Geometry: final body of the model. Coordinates: model frame, mm. Face numbers are marked on the shaded views. A direction names the side the tool comes from. Round coordinates to 2 decimals unless told otherwise and drop trailing zeros. Write each loop counter-clockwise with the first axis right and the second up, starting at its lowest first coordinate (ties: lowest second). Pieces come first, ordered by that corner, then holes. Notation, with made-up numbers: M 48.5,48 L 53.5,48 A19 cw 53.5,70 Z; hole C 67.5,5 d5. An arc over 180 degrees is marked long. Put each result on its own line as item: value. Start each with the question number.
Autodesk Inventor part; units mm, degrees
ref_plane "YZ Plane" through (0, 0, 0) normal (1, 0, 0) x (0, 1, 0)
ref_plane "XZ Plane" through (0, 0, 0) normal (0, 1, 0) x (-1, 0, 0)
ref_plane "XY Plane" through (0, 0, 0) normal (0, 0, 1) x (1, 0, 0)
sketch "Sketch1" plane through (0, 0, 0) normal (0, 0, 1) x (1, 0, 0)
  circle A0 centre (0, 0) radius 14.2875
  circle A1 centre (0, 0) radius 6.35
  dimension "d0" = 28.575
  dimension "d1" = 12.7
extrude "Extrusion1" add sketch "Sketch1" along normal blind 7.7724
sketch "Sketch2" plane through (0, 0, 0) normal (0, 0, -1) x (-1, 0, 0)
  circle A0 centre (0, 0) radius 15.5575
  circle A1 centre (0, 0) radius 14.2875
  circle A2 centre (0, 0) radius 6.35
  dimension "d4" = 31.115
  dimension "d5" = 12.7
extrude "Extrusion2" add sketch "Sketch2" along normal blind 1.524 contours A0 | A1
properties part number "bearing"
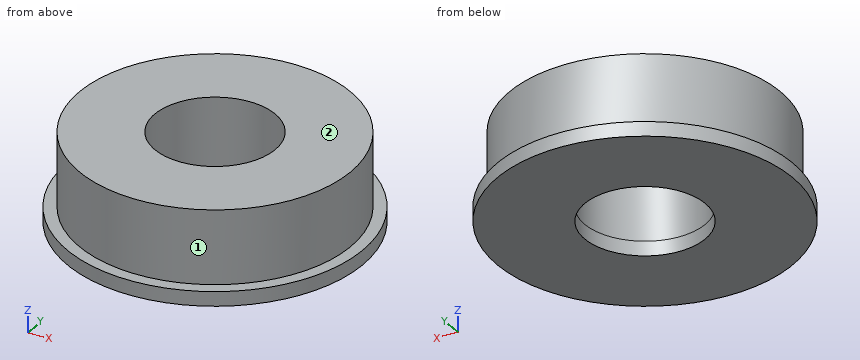
1) First-contact query: pin 1 (7.5 mm diameter, centred on x = 0, y = 0, fed in from +Z); pin 2 (14.5 mm diameter, centred on x = 0, y = 0, fed in from +Z); pin 3 (3 mm diameter, centred on y = -4.5, z = 2, fed in from +X). Flat tips, straight axial feed; report the tip coordinate or a pass-through.
2) Section A-A, the plane y = 0. Output: boundary loops of the cut face in (x, z).
3) Section D-D, the plane x = -9. Output: boundary loops of the cut face in (y, z), and give its area (3 significant figures).
4) Ray query, probe 1 along X at (y, z) = (-5.5, 2.5); probe 2 along Y at (x, z) = (3.5, 1.75); probe 3 along Y at (x, z) = (-3.5, -0.5). Return the intervals inside material, ascending.
5) Access query for the marked faces 1 and 2. Directions: +Z, -Z, +X, -X, +Y, -Y. A direction counts if a zero-diameter tool reaches every point of the face in a straight line with its end or side. Return the directions, or none.
Solved:
1. pin 1: passes through
1. pin 2: stops at z = 7.77
1. pin 3: stops at x = 13.97
2. outline: M -15.56,-1.52 L -6.35,-1.52 L -6.35,7.77 L -14.29,7.77 L -14.29,0 L -15.56,0 Z; M 6.35,-1.52 L 15.56,-1.52 L 15.56,0 L 14.29,0 L 14.29,7.77 L 6.35,7.77 Z
3. outline: M -12.69,-1.52 L 12.69,-1.52 L 12.69,0 L 11.1,0 L 11.1,7.77 L -11.1,7.77 L -11.1,0 L -12.69,0 Z
3. area: 211 mm2
4. probe 1: x = -13.19 to -3.17, 3.17 to 13.19
4. probe 2: y = -13.85 to -5.3, 5.3 to 13.85
4. probe 3: y = -15.16 to -5.3, 5.3 to 15.16
5. face 1: +Z
5. face 2: +Z, +X, -X, +Y, -Y
